from build123d import *

# Parameters (mm, degrees)
SKETCH_1_R          = 12.5
EXTRUDE_1_DEPTH     = 8
SKETCH_2_R          = 15
EXTRUDE_2_DEPTH     = 30
SKETCH_3_R          = 10
CUT_EXTRUDE_1_DEPTH = 15
SKETCH_5_R          = 12.5
EXTRUDE_3_DEPTH     = 3
SKETCH_6_R          = 12.5
SKETCH_6_R_2        = 12.1
CUT_EXTRUDE_2_DEPTH = 1.2
EXTRUDE_START       = 2
SKETCH_9_R          = 15
SKETCH_9_R_2        = 12.5
EXTRUDE_4_DEPTH     = 2
SKETCH_12_R         = 1.5
CUT_EXTRUDE_6_DEPTH = 47.162755705
SKETCH_13_R         = 6
CUT_EXTRUDE_7_DEPTH = 20
SKETCH_14_W         = 23.536155202
SKETCH_14_H         = 8
CUT_EXTRUDE_8_DEPTH = 20
FILLET_1_R          = 3


with BuildPart() as part:
    # 草图1 → 凸台-拉伸1 (new body)
    with BuildSketch(Plane.XY):
        Circle(SKETCH_1_R)
    extrude(amount=EXTRUDE_1_DEPTH)

    # 草图2 → 凸台-拉伸2 (add)
    with BuildSketch(Plane(origin=(0, 0, 0), x_dir=(-1, 0, 0), z_dir=(0, 0, -1))):
        Circle(SKETCH_2_R)
    extrude(amount=EXTRUDE_2_DEPTH)

    # 草图3 → 切除-拉伸1 (cut, symmetric)
    with BuildSketch(Plane(origin=(0, 0, 0), x_dir=(0, 0, -1), z_dir=(1, 0, 0))):
        with Locations((15, 0)):
            Circle(SKETCH_3_R)
    extrude(amount=CUT_EXTRUDE_1_DEPTH, both=True, mode=Mode.SUBTRACT)

    # 草图5 → 凸台-拉伸3 (add)
    with BuildSketch(Plane.XY.offset(8)):
        Circle(SKETCH_5_R)
    extrude(amount=EXTRUDE_3_DEPTH)

    # 草图6 → 切除-拉伸2 (cut)
    with BuildSketch(Plane.XY.offset(7)):
        Circle(SKETCH_6_R)
        Circle(SKETCH_6_R_2, mode=Mode.SUBTRACT)
    extrude(amount=CUT_EXTRUDE_2_DEPTH, mode=Mode.SUBTRACT)

    # 草图9 → 凸台-拉伸4 (add)
    with BuildSketch(Plane(origin=(0, 0, 0), x_dir=(-1, 0, 0), z_dir=(0, 0, -1)).offset(EXTRUDE_START)):
        Circle(SKETCH_9_R)
        with Locations(Location((0, 0, 0), (0, 0, 180))):
            Circle(SKETCH_9_R_2, mode=Mode.SUBTRACT)
    extrude(amount=-EXTRUDE_4_DEPTH)

    # 草图12 → 切除-拉伸6 (cut, through all)
    with BuildSketch(Plane.XY.offset(11)):
        with Locations((6.717514421, 6.717514421)):
            Circle(SKETCH_12_R)
        with Locations((6.717514421, -6.717514421)):
            Circle(SKETCH_12_R)
        with Locations((-6.717514421, -6.717514421)):
            Circle(SKETCH_12_R)
        with Locations((-6.717514421, 6.717514421)):
            Circle(SKETCH_12_R)
    extrude(amount=-CUT_EXTRUDE_6_DEPTH, mode=Mode.SUBTRACT)

    # 草图13 → 切除-拉伸7 (cut)
    with BuildSketch(Plane.XY.offset(11)):
        Circle(SKETCH_13_R)
    extrude(amount=-CUT_EXTRUDE_7_DEPTH, mode=Mode.SUBTRACT)

    # 草图14 → 切除-拉伸8 (cut)
    with BuildSketch(Plane.XY.offset(11)):
        with Locations((-12.5, 0)):
            Rectangle(SKETCH_14_W, SKETCH_14_H)
    extrude(amount=-CUT_EXTRUDE_8_DEPTH, mode=Mode.SUBTRACT)

    # 圆角1
    fillet_1_edges = [part.edges().sort_by_distance(p)[0] for p in [
        (15, 0, -30),
    ]]
    fillet(fillet_1_edges, radius=FILLET_1_R)


solid = part.part
Geometry check sheet. Reference: the model listing, model coordinates, mm. A direction names the side the tool comes from. Round coordinates to 2 decimals unless told otherwise and drop trailing zeros. Loops run counter-clockwise (first coordinate to the right, second up) from the corner with the lowest first, then second, coordinate; pieces in that order, holes last.
Item 1: Cross-section at C-C on x = 0. Record the boundary of the cut face in (y, z).
Item 2: Gauge pin test, flat ends, axial feed: pin 1 (3 mm diameter, centred on x = -10, z = 6, fed in from -Y); pin 2 (3 mm diameter, centred on x = -11, z = 0.5, fed in from +Y); pin 3 (7 mm diameter, centred on x = 0, y = 0, fed in from +Z); pin 4 (1.8 mm diameter, centred on x = -6.72, y = -6.72, fed in from +Z). Record the tip position at first contact, or that the pin passes through.
Item 3: Cross-section at B-B on z = -23. Record the boundary of the cut face in (x, y).
Item 4: Thickness scan on line 1 (Z direction, x = 8, y = 0); line 2 (X direction, y = 8, z = -2); line 3 (Y direction, x = 1.5, z = 8). Record the ranges inside material, lowest first.
Item 5: Mould release check, pull along X, two halves, no side actions. Record for faces 1 (the cylindrical face through (12.49, -0.49, 3.45)), 2 (the flat face through (0, 0, -30)), 3 (the cylindrical face through (7.41, -8.05, 0.99)), 4 (the cylindrical face through (-6.03, -8.05, 0.99)): pulls with the +X half, pulls with the -X half, needs draft (parallel to the pull), parting line crosses it, or undercut.
Item 6: Cross-section at D-D on z = 3. Record the boundary of the cut face in (x, y), then the cut area to 3 significant figures.
Item 7: Access from +Z, -Z, +X, -X, +Y, -Y to the whole of each face (thin tool, end or side, straight path). Record for faces 5 (the flat face through (2.1, 12.1, 8.2)), 6 (the cylindrical face through (12.49, -0.49, 9.58)), 7 (the cylindrical face through (-7.043, -8.182, -26.318)).
Item 8: Cross-section at A-A on y = 0. Record the boundary of the cut face in (x, z), then the cut area to 3 significant figures.
Answer sheet:
1. outline: (-15, -27) arc R3 ccw to (-12, -30) - (12, -30) arc R3 ccw to (15, -27) - (15, 0) - (12.5, 0) - (12.5, 7) - (12.1, 7) - (12.1, 8.2) - (12.5, 8.2) - (12.5, 11) - (6, 11) - (6, -7) arc R10 cw (long way) to (-6, -7) - (-6, 11) - (-12.5, 11) - (-12.5, 8.2) - (-12.1, 8.2) - (-12.1, 7) - (-12.5, 7) - (-12.5, 0) - (-15, 0) - close
2. pin 1: stops at y = -9.17
2. pin 2: stops at y = 11.54
2. pin 3: stops at z = -24.37
2. pin 4: passes through
3. outline: (-13.75, -6) arc R15 ccw to (13.75, -6) - (8.03, -6) arc R1.5 cw (long way) to (5.4, -6) - (-5.4, -6) arc R1.5 cw (long way) to (-8.03, -6) - close; (-13.75, 6) - (-8.03, 6) arc R1.5 cw (long way) to (-5.4, 6) - (5.4, 6) arc R1.5 cw (long way) to (8.03, 6) - (13.75, 6) arc R15 ccw to start
4. line 1: z = -30 to -25, -5 to 11
4. line 2: x = -12.69 to -7.5, -5.94 to 5.94, 7.5 to 12.69
4. line 3: y = -12.01 to -5.81, 5.81 to 12.01
5. face 1: parting line crosses it
5. face 2: needs draft
5. face 3: undercut
5. face 4: undercut
6. outline: (-11.84, -4) arc R12.5 ccw (long way) to (-11.84, 4) - (-4.47, 4) arc R6 cw (long way) to (-4.47, -4) - close; hole circle Ø3 at (-6.72, -6.72); hole circle Ø3 at (-6.72, 6.72); hole circle Ø3 at (6.72, -6.72); hole circle Ø3 at (6.72, 6.72)
6. area: 295 mm2
7. face 5: none
7. face 6: +Z
7. face 7: +Z, -Z
8. outline: (-15, -27) arc R3 ccw to (-12, -30) - (12, -30) arc R3 ccw to (15, -27) - (15, -25) - (-15, -25) - close; (6, -5) - (15, -5) - (15, 0) - (12.5, 0) - (12.5, 7) - (12.1, 7) - (12.1, 8.2) - (12.5, 8.2) - (12.5, 11) - (6, 11) - close
8. area: 262 mm2
